Model file for the job. Use its own axes, mm. A direction names the side the tool comes from. Coordinates: 2 decimals unless noted, no trailing zeros. Order: outer loops, then holes, each group sorted by start corner. A loop starts at its lowest first (then second) coordinate and runs counter-clockwise, first axis right, second up.
Autodesk Inventor part; units mm, degrees
ref_plane "YZ Plane" through (0, 0, 0) normal (1, 0, 0) x (0, 1, 0)
ref_plane "XZ Plane" through (0, 0, 0) normal (0, 1, 0) x (-1, 0, 0)
ref_plane "XY Plane" through (0, 0, 0) normal (0, 0, 1) x (1, 0, 0)
sketch "Sketch1" plane through (0, 0, 0) normal (0, 0, 1) x (1, 0, 0)
  circle A0 centre (0, 0) radius 19.05
  dimension "d0" = 38.1
extrude "Extrusion1" add sketch "Sketch1" along normal blind 152.4
sketch "Sketch2" plane through (0, 0, 152.4) normal (0, 0, 1) x (1, 0, 0)
  circle A0 centre (0, 0) radius 3.175
  dimension "d3" = 6.35
extrude "Extrusion2" add sketch "Sketch2" along normal blind 6.35
sketch "Sketch3" plane through (0, 0, 0) normal (0, 0, -1) x (-1, 0, 0)
  circle A0 centre (0, 0) radius 3.175
  circle A1 centre (0, 0) radius 3.175
extrude "Extrusion3" add sketch "Sketch3" along normal blind 6.35
properties part number "Roller"
Q1. Probe line 1 (Z direction, x = -5, y = -15); line 2 (Y direction, x = 0, z = 49); line 3 (Y direction, x = 12.5, z = 54). List the from-to ranges inside material, lowest first.
Established:
line 1: z = 0 to 152.4
line 2: y = -19.05 to 19.05
line 3: y = -14.38 to 14.38
Q2. Mould opens along X. For faces 1 (the face through (0.69, 3.1, -3.13)), 2 (the face through (0, 0, 158.75)) say: pulls with the +X half, pulls with the -X half, needs draft (parallel to the pull), parting line crosses it, or undercut.
Established:
face 1: parting line crosses it
face 2: needs draft
Q3. Cut at A-A, the plane x = 0. List the corners of the cut face in (y, z) (3 decimals).
Established:
outline: (-19.05, 0) - (-3.175, 0) - (-3.175, -6.35) - (3.175, -6.35) - (3.175, 0) - (19.05, 0) - (19.05, 152.4) - (3.175, 152.4) - (3.175, 158.75) - (-3.175, 158.75) - (-3.175, 152.4) - (-19.05, 152.4) - close
Q4. Cut at D-D, the plane x = -12. List the corners of the cut face in (y, z), plus the area to 3 significant figures.
Established:
outline: (-14.8, 0) - (14.8, 0) - (14.8, 152.4) - (-14.8, 152.4) - close
area: 4,510 mm2
Q5. Drop flat-ended pins along their axis: P1, Ø8, axis at y = -8.5, z = 125.5, coming from the -X side; P2, Ø2, axis at y = -9.5, z = 39.5, coming from the +X side; P3, Ø11.5, axis at x = -8.5, y = 4.5, coming from the -Z side. Give the stop position or say it passes through.
Established:
P1: stops at x = -18.51
P2: stops at x = 17.05
P3: stops at z = 0
Q6. Cut at C-C, the plane z = 45. List the corners of the cut face in (x, y).
Established:
outline: circle Ø38.1 at (0, 0)
Q7. Which spindle directions (+Z, -Z, +X, -X, +Y, -Y) get a long thin tool onto all of the face, cutting with end or side? Do faces 3 (the face through (-15.12, 11.59, 75.13)), 4 (the face through (-0.69, 3.1, 155.53)). Say none if no direction does.
Established:
face 3: +Z, -Z
face 4: +Z
